from build123d import *

# Parameters (mm, degrees)
SKETCH1_W           = 170.9
SKETCH1_H           = 120
BOSS_EXTRUDE1_DEPTH = 5.9
SKETCH2_W           = 5.9
SKETCH2_H           = 10
CUT_EXTRUDE1_DEPTH  = 6.9
CUT_EXTRUDE4_REACH  = 7.9
SKETCH5_R           = 2.05


with BuildPart() as part:
    # Sketch1 → Boss-Extrude1 (new body)
    with BuildSketch(Plane.XY):
        Rectangle(SKETCH1_W, SKETCH1_H)
    extrude(amount=BOSS_EXTRUDE1_DEPTH)

    # Sketch2 → Cut-Extrude1 (cut, through all)
    with BuildSketch(Plane.XY.offset(5.9)):
        with Locations((82.5, 25)):
            Rectangle(SKETCH2_W, SKETCH2_H)
        with Locations((82.5, -25)):
            Rectangle(SKETCH2_W, SKETCH2_H)
        with Locations((-82.5, -25)):
            Rectangle(SKETCH2_W, SKETCH2_H)
        with Locations((-82.5, 25)):
            Rectangle(SKETCH2_W, SKETCH2_H)
    extrude(amount=-CUT_EXTRUDE1_DEPTH, mode=Mode.SUBTRACT)

    # Sketch5 → Cut-Extrude4 (cut, up to next)
    with BuildSketch(Plane.XY.offset(5.9), mode=Mode.PRIVATE) as cut_extrude4_sk1:
        with Locations((-79.55, 30)):
            Circle(SKETCH5_R)
    cut_extrude4_tool1 = extrude(cut_extrude4_sk1.sketch, amount=-CUT_EXTRUDE4_REACH, mode=Mode.PRIVATE) & part.part
    add(cut_extrude4_tool1.solids().sort_by_distance((-79.55, 30, 5.9))[0], mode=Mode.SUBTRACT)
    # Sketch5 → Cut-Extrude4 (cut, up to next)
    with BuildSketch(Plane.XY.offset(5.9), mode=Mode.PRIVATE) as cut_extrude4_sk2:
        with Locations((-79.55, 20)):
            Circle(SKETCH5_R)
    cut_extrude4_tool2 = extrude(cut_extrude4_sk2.sketch, amount=-CUT_EXTRUDE4_REACH, mode=Mode.PRIVATE) & part.part
    add(cut_extrude4_tool2.solids().sort_by_distance((-79.55, 20, 5.9))[0], mode=Mode.SUBTRACT)
    # Sketch5 → Cut-Extrude4 (cut, up to next)
    with BuildSketch(Plane.XY.offset(5.9), mode=Mode.PRIVATE) as cut_extrude4_sk3:
        with Locations((-79.55, -20)):
            Circle(SKETCH5_R)
    cut_extrude4_tool3 = extrude(cut_extrude4_sk3.sketch, amount=-CUT_EXTRUDE4_REACH, mode=Mode.PRIVATE) & part.part
    add(cut_extrude4_tool3.solids().sort_by_distance((-79.55, -20, 5.9))[0], mode=Mode.SUBTRACT)
    # Sketch5 → Cut-Extrude4 (cut, up to next)
    with BuildSketch(Plane.XY.offset(5.9), mode=Mode.PRIVATE) as cut_extrude4_sk4:
        with Locations((-79.55, -30)):
            Circle(SKETCH5_R)
    cut_extrude4_tool4 = extrude(cut_extrude4_sk4.sketch, amount=-CUT_EXTRUDE4_REACH, mode=Mode.PRIVATE) & part.part
    add(cut_extrude4_tool4.solids().sort_by_distance((-79.55, -30, 5.9))[0], mode=Mode.SUBTRACT)
    # Sketch5 → Cut-Extrude4 (cut, up to next)
    with BuildSketch(Plane.XY.offset(5.9), mode=Mode.PRIVATE) as cut_extrude4_sk5:
        with Locations((79.55, -20)):
            Circle(SKETCH5_R)
    cut_extrude4_tool5 = extrude(cut_extrude4_sk5.sketch, amount=-CUT_EXTRUDE4_REACH, mode=Mode.PRIVATE) & part.part
    add(cut_extrude4_tool5.solids().sort_by_distance((79.55, -20, 5.9))[0], mode=Mode.SUBTRACT)
    # Sketch5 → Cut-Extrude4 (cut, up to next)
    with BuildSketch(Plane.XY.offset(5.9), mode=Mode.PRIVATE) as cut_extrude4_sk6:
        with Locations((79.55, -30)):
            Circle(SKETCH5_R)
    cut_extrude4_tool6 = extrude(cut_extrude4_sk6.sketch, amount=-CUT_EXTRUDE4_REACH, mode=Mode.PRIVATE) & part.part
    add(cut_extrude4_tool6.solids().sort_by_distance((79.55, -30, 5.9))[0], mode=Mode.SUBTRACT)
    # Sketch5 → Cut-Extrude4 (cut, up to next)
    with BuildSketch(Plane.XY.offset(5.9), mode=Mode.PRIVATE) as cut_extrude4_sk7:
        with Locations((79.55, 20)):
            Circle(SKETCH5_R)
    cut_extrude4_tool7 = extrude(cut_extrude4_sk7.sketch, amount=-CUT_EXTRUDE4_REACH, mode=Mode.PRIVATE) & part.part
    add(cut_extrude4_tool7.solids().sort_by_distance((79.55, 20, 5.9))[0], mode=Mode.SUBTRACT)
    # Sketch5 → Cut-Extrude4 (cut, up to next)
    with BuildSketch(Plane.XY.offset(5.9), mode=Mode.PRIVATE) as cut_extrude4_sk8:
        with Locations((79.55, 30)):
            Circle(SKETCH5_R)
    cut_extrude4_tool8 = extrude(cut_extrude4_sk8.sketch, amount=-CUT_EXTRUDE4_REACH, mode=Mode.PRIVATE) & part.part
    add(cut_extrude4_tool8.solids().sort_by_distance((79.55, 30, 5.9))[0], mode=Mode.SUBTRACT)


solid = part.part
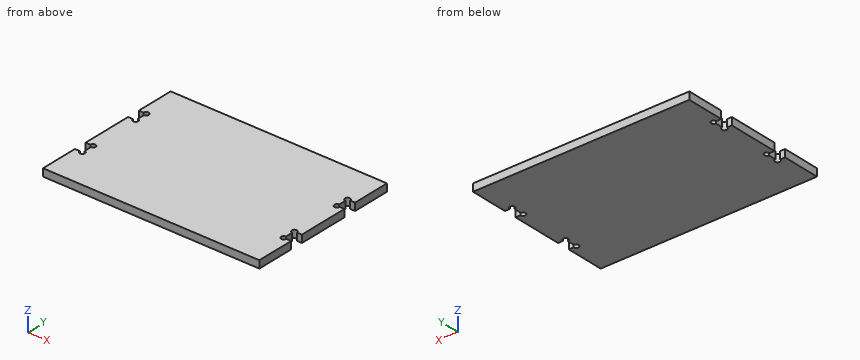
Can you work these out from the model? Positions are in its coordinate system, mm. Coordinates: 2 decimals unless noted, no trailing zeros. Order: outer loops, then holes, each group sorted by start corner. A loop starts at its lowest first (then second) coordinate and runs counter-clockwise, first axis right, second up. Notation, with made-up numbers: (-14, -27) -> (-7, -27) arc R21 cw to (-7, -9) -> close; hole circle Ø9 at (-29, 58). An arc over 180 degrees is marked (long way). Use one line per item in the form item = value.
Q1. Will these pins go through, and if not, where does the flat tip stop? P1, Ø3, axis at y = -26.5, z = 4, coming from the -X side; P2, Ø3, axis at y = 26.5, z = 4.5, coming from the +X side; P3, Ø3.5, axis at x = 79.55, y = 30, coming from the -Z side; P4, Ø1.5, axis at y = 21, z = 1, coming from the +X side.
From the geometry:
P1 = -79.55
P2 = 79.55
P3 = through
P4 = 78.48
Q2. I need wall thicknesses on L1, parallel to X at y = 26, z = 1.6. Which ranges of the line are inside material? Lowest first, please.
From the geometry:
L1 = -79.55 to 79.55
Q3. Imagine slicing it at A-A, the plane z = 1.3. List the corners of the cut face in (x, y) for me.
From the geometry:
outline = (-85.45, -60) -> (85.45, -60) -> (85.45, -30) -> (81.6, -30) arc R2.05 cw (long way) to (79.55, -27.95) -> (79.55, -22.05) arc R2.05 cw (long way) to (81.6, -20) -> (85.45, -20) -> (85.45, 20) -> (81.6, 20) arc R2.05 cw (long way) to (79.55, 22.05) -> (79.55, 27.95) arc R2.05 cw (long way) to (81.6, 30) -> (85.45, 30) -> (85.45, 60) -> (-85.45, 60) -> (-85.45, 30) -> (-81.6, 30) arc R2.05 cw (long way) to (-79.55, 27.95) -> (-79.55, 22.05) arc R2.05 cw (long way) to (-81.6, 20) -> (-85.45, 20) -> (-85.45, -20) -> (-81.6, -20) arc R2.05 cw (long way) to (-79.55, -22.05) -> (-79.55, -27.95) arc R2.05 cw (long way) to (-81.6, -30) -> (-85.45, -30) -> close
